```python
from build123d import *

# Parameters (mm, degrees)
SKETCH1_W           = 250
SKETCH1_H           = 100
BOSS_EXTRUDE1_DEPTH = 33
CHAMFER1_SIZE       = 35
SKETCH2_R           = 20
CUT_EXTRUDE1_DEPTH  = 35
SKETCH3_R           = 15
CUT_EXTRUDE2_DEPTH  = 33
LPATTERN1_COUNT     = 2
LPATTERN1_PITCH     = 180


with BuildPart() as part:
    # Sketch1 → Boss-Extrude1 (new body)
    with BuildSketch(Plane.XY):
        with Locations((14.758290847, 1.860150752)):
            Rectangle(SKETCH1_W, SKETCH1_H)
    extrude(amount=BOSS_EXTRUDE1_DEPTH)

    # Chamfer1
    chamfer1_edges = [part.edges().sort_by_distance(p)[0] for p in [
        (-110.241709153, 51.860150752, 16.5),
        (139.758290847, 51.860150752, 16.5),
        (139.758290847, -48.139849248, 16.5),
        (-110.241709153, -48.139849248, 16.5),
    ]]
    chamfer(chamfer1_edges, length=CHAMFER1_SIZE)

    # Sketch2 → Cut-Extrude1 (cut)
    with BuildSketch(Plane.XY.offset(33)):
        with Locations((14.758290847, 1.860150752)):
            Circle(SKETCH2_R)
    extrude(amount=-CUT_EXTRUDE1_DEPTH, mode=Mode.SUBTRACT)

    # Sketch3 → Cut-Extrude2 (cut)
    with BuildSketch(Plane.XY.offset(33)):
        with Locations((104.758290847, 1.860150752)):
            Circle(SKETCH3_R)
    cut_extrude2 = extrude(amount=-CUT_EXTRUDE2_DEPTH, mode=Mode.SUBTRACT)

    # LPattern1: Cut-Extrude2 ×2
    with Locations(*[(-i * LPATTERN1_PITCH, 0, 0) for i in range(1, LPATTERN1_COUNT)]):
        add(cut_extrude2, mode=Mode.SUBTRACT)


solid = part.part
```
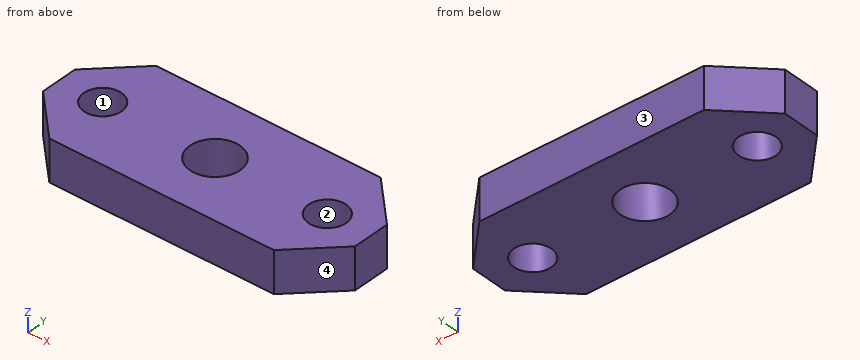
Geometry: final body of the model. Coordinates: model frame, mm. Face numbers are marked on the shaded views. Give positions to 0.01 mm unless a question says otherwise; leave off trailing zeros. Loops run counter-clockwise (first coordinate to the right, second up) from the corner with the lowest first, then second, coordinate; pieces in that order, holes last. Notation, with made-up numbers: (59.5, 54.25) - (75.5, 54.25) arc R15 cw to (75.5, 67.25) - close; hole circle Ø9 at (22, -12.75). An arc over 180 degrees is marked (long way). Answer as CSV lines item,"result". Start each with the question number.
(1) Section query A-A (x = -64). Output: boundary loops of the cut face in (y, z), and give its area (3 significant figures).
(2) Mould query, pull axis X, two halves, no side actions, for the marked faces 1, 2, 3 and 4. Classes: +X half, -X half, draft (parallel to the pull), parting line (faces both ways), or undercut.
(3) Section query D-D (x = 31.5). Output: boundary loops of the cut face in (y, z).
(4) Pin query (flat end, axial travel): P1, Ø12, axis at y = -34.5, z = 17, coming from the +X side; P2, Ø2, axis at y = 33, z = 10, coming from the +X side; P3, Ø10, axis at y = 21.5, z = 22.5, coming from the -X side. Return the tip coordinate at first contact, or that it passes through.
(5) Ray query, line 1 along X through (y, z) = (3, 31); line 2 along X through (y, z) = (11.5, 28.5); line 3 along Y through (x, z) = (92, 14). Return the intervals inside material, ascending. Write a range as [from, to].
(6) Section query B-B (y = -6). Output: boundary loops of the cut face in (x, z), and give its area (3 significant figures).
(7) Section query C-C (z = 27). Output: boundary loops of the cut face in (x, y).
Worked answers:
1,outline,"(-48.14, 0) - (-8.07, 0) - (-8.07, 33) - (-48.14, 33) - close; (11.79, 0) - (51.86, 0) - (51.86, 33) - (11.79, 33) - close"
1,area,"2,640 mm^2"
2,face 1,"undercut"
2,face 2,"undercut"
2,face 3,"draft"
2,face 4,"+X half"
3,outline,"(-48.14, 0) - (-9.08, 0) - (-9.08, 33) - (-48.14, 33) - close; (12.8, 0) - (51.86, 0) - (51.86, 33) - (12.8, 33) - close"
4,P1,"stops at x = 124.4"
4,P2,"stops at x = 124.62"
4,P3,"stops at x = -110.24"
5,line 1,"x = [-110.24, -90.2], [-60.29, -5.21], [34.73, 89.8], [119.71, 139.76]"
5,line 2,"x = [-110.24, -86.73], [-63.75, -2.77], [32.28, 93.27], [116.25, 139.76]"
5,line 3,"y = [-48.14, -6.03], [9.75, 51.86]"
6,outline,"(-110.24, 0) - (-88.02, 0) - (-88.02, 33) - (-110.24, 33) - close; (-62.47, 0) - (-3.63, 0) - (-3.63, 33) - (-62.47, 33) - close; (33.15, 0) - (91.98, 0) - (91.98, 33) - (33.15, 33) - close; (117.53, 0) - (139.76, 0) - (139.76, 33) - (117.53, 33) - close"
6,area,"5,350 mm^2"
7,outline,"(-110.24, -13.14) - (-75.24, -48.14) - (104.76, -48.14) - (139.76, -13.14) - (139.76, 16.86) - (104.76, 51.86) - (-75.24, 51.86) - (-110.24, 16.86) - close; hole circle Ø30 at (-75.24, 1.86); hole circle Ø40 at (14.76, 1.86); hole circle Ø30 at (104.76, 1.86)"
